from build123d import *

# Parameters (mm, degrees)
F1_DEPTH = 5
F3_DEPTH = 25


with BuildPart() as f1:
    # F0 (on Top) → F1 (new body)
    with BuildSketch(Plane.XY):
        with BuildLine():
            Line((-23.5, 8.5), (-23.5, 0))
            Line((-23.5, 0), (23.5, 0))
            Line((23.5, 0), (23.5, 6.5))
            ThreePointArc((23.5, 6.5), (0.2962107176, 14.4609518625), (-23.5, 8.5))
        make_face()
    extrude(amount=F1_DEPTH)

    # F2 (on face) → F3 (cut)
    with BuildSketch(Plane.XY.offset(5)):
        with BuildLine():
            Line((-23.5, 0), (-22.5, 0))
            Line((-22.5, 0), (-22.5, 3))
            Line((-22.5, 3), (-19.5, 3))
            ThreePointArc((-19.5, 3), (-18.5, 4), (-19.5, 5))
            ThreePointArc((-19.5, 5), (-22.1575364532, 5.9985297678), (-23.5, 8.5))
            Line((-23.5, 8.5), (-23.5, 0))
        make_face()
        with BuildLine():
            Line((-8.5, 3), (-8.5, 0))
            Line((-8.5, 0), (6.5, 0))
            Line((6.5, 0), (6.5, 3))
            Line((6.5, 3), (10.4063445255, 3))
            ThreePointArc((10.4063445255, 3), (11.390316995, 3.8216795603), (10.7572693324, 4.9364036415))
            ThreePointArc((10.7572693324, 4.9364036415), (-1, 7.0671151221), (-12.7572693324, 4.9364036415))
            ThreePointArc((-12.7572693324, 4.9364036415), (-13.390316995, 3.8216795603), (-12.4063445255, 3))
            Line((-12.4063445255, 3), (-8.5, 3))
        make_face()
        with BuildLine():
            Line((23.5, 0), (23.5, 6.5))
            ThreePointArc((23.5, 6.5), (20.8467428507, 4.363028597), (17.5, 5))
            ThreePointArc((17.5, 5), (16.5, 4), (17.5, 3))
            Line((17.5, 3), (20.5, 3))
            Line((20.5, 3), (20.5, 0))
            Line((20.5, 0), (23.5, 0))
        make_face()
    extrude(amount=-F3_DEPTH, mode=Mode.SUBTRACT)

    # F6: sweep along a path in F6_path
    with BuildLine(Plane(origin=(-23.5, 8.5, 0), x_dir=(0, 1, 0), z_dir=(0, 0, 1))) as f6_path:
        ThreePointArc((0, 0), (5.9609518625, -23.7962107176), (-2, -47))
    # F5 (on face) → F6 (sweep, cut)
    with BuildSketch(Plane(origin=(-13.7022180635, -8.0915495232, 0), x_dir=(0.5084863558, -0.8610700471, 0), z_dir=(-0.8610700471, -0.5084863558, 0))):
        Polygon((-19.2685247607, 5), (-19.2685247607, 1), (-17.2685247607, 5), align=None)
    sweep(path=f6_path.line, mode=Mode.SUBTRACT)


solid = f1.part
Check sheet for the modelled part. Datum: model origin and axes. Units: mm. A direction names the side the tool comes from. Round coordinates to 2 decimals unless told otherwise and drop trailing zeros. Loops run counter-clockwise (first coordinate to the right, second up) from the corner with the lowest first, then second, coordinate; pieces in that order, holes last. Notation, with made-up numbers: M -31.5,-15.5 L -19.5,-15.5 A23 ccw -19.5,16.5 Z; hole C -5.5,75 d8. An arc over 180 degrees is marked long. One line per item, written item: value.
(1) Release check for a two-part mould opening along Y. For faces 5 (the face through (-21, 3, 3)), 6 (the face through (-0.102, 13.017, 3.917)), 7 (the face through (-10, 3, 3)), 8 (the face through (-16, 0, 2)) record: +Y half, -Y half, draft (parallel to the pull), parting line (faces both ways), or undercut.
Computed values:
face 5: undercut
face 6: +Y half
face 7: undercut
face 8: -Y half
(2) Access from +Z, -Z, +X, -X, +Y, -Y to the whole of each face (thin tool, end or side, straight path). Record for faces 1 (the face through (-22.127, 5.972, 2.535)), 2 (the face through (8, 3, 3)), 3 (the face through (19, 3, 3)), 4 (the face through (-22.5, 1, 3)).
Computed values:
face 1: +Z, -Z, -X
face 2: +Z, -Z
face 3: +Z, -Z, +X
face 4: +Z, -Z, -X, -Y
(3) Sectioned sample at B-B, the plane z = 2.55. Record the cut outline in (x, y).
Computed values:
outline: M -23.5,8.5 A4.04 ccw -19.5,5 A1 cw -19.5,3 L -22.5,3 L -22.5,0 L -8.5,0 L -8.5,3 L -12.41,3 A1 cw -12.76,4.94 A33.5 cw 10.76,4.94 A1 cw 10.41,3 L 6.5,3 L 6.5,0 L 20.5,0 L 20.5,3 L 17.5,3 A1 cw 17.5,5 A4.06 ccw 23.5,6.5 L 23.05,5.87 A42.41 ccw -23.11,7.83 Z
(4) Sectioned sample at A-A, the plane y = 3.5. Record the cut outline in (x, z), then the cut area to 3 significant figures.
Computed values:
outline: M -18.63,0 L -13.27,0 L -13.27,5 L -18.63,5 Z; M 11.27,0 L 16.63,0 L 16.63,5 L 11.27,5 Z
area: 53.6 mm^2
(5) Thickness scan on line 1 (Y direction, x = -11, z = 0.7); line 2 (Z direction, x = 18, y = 8); line 3 (X direction, y = 1.5, z = 3.9). Record the ranges inside material, lowest first.
Computed values:
line 1: y = 0 to 3, 5.54 to 13.45
line 2: z = 0 to 4.24
line 3: x = -22.5 to -8.5, 6.5 to 20.5
(6) Depth check by flat-ended pin: pin 1 Ø1 at (y, z) = (9, 3) entering from +X; pin 2 Ø1.5 at (y, z) = (1.5, 3.5) entering from -X; pin 3 Ø1.5 at (y, z) = (2, 2.5) entering from +X. Enter the tip coordinate at first touch or a pass-through.
Computed values:
pin 1: stops at x = 18.52
pin 2: stops at x = -22.5
pin 3: stops at x = 20.5
